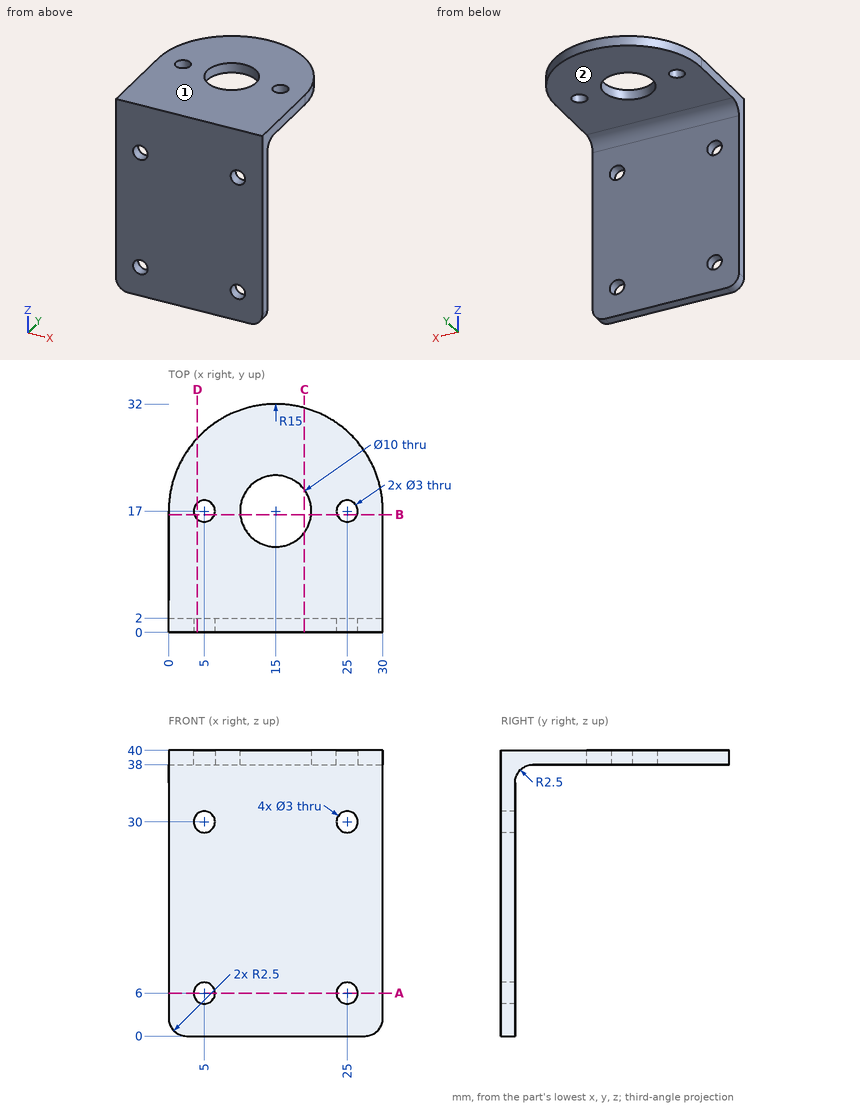
Input: dimensioned drawing with shaded views. Units: mm. Origin: part minimum x, y, z. A direction names the side the tool comes from. Give positions to 0.01 mm unless a question says otherwise; leave off trailing zeros. Loops run counter-clockwise (first coordinate to the right, second up) from the corner with the lowest first, then second, coordinate; pieces in that order, holes last. Notation, with made-up numbers: (4.5, -36.75) - (56.5, -36.75) arc R27 ccw to (56.5, -0.75) - close; hole circle Ø6 at (83, 60.25). An arc over 180 degrees is marked (long way). Answer as CSV lines item,"result". Start each with the question number.
(1) Section query B-B (y = 16.5). Output: boundary loops of the cut face in (x, z), and give its area (3 significant figures).
(2) Pin query (flat end, axial travel): P1, Ø4, axis at x = 4, y = 22, coming from the -Z side. Return the tip coordinate at first contact, or that it passes through.
(3) Reachability of the marked faces 1 and 2 from +Z, -Z, +X, -X, +Y, -Y: full face, straight path, thin tool, end or side. Return the list, or none.
(4) Ray query, line 1 along Z through (x, y) = (5, 1.5); line 2 along Y through (x, z) = (11.5, 8.5); line 3 along Z through (x, y) = (1.5, 5). Return the intervals inside material, ascending. Write a range as [from, to].
(5) Section query A-A (z = 6). Output: boundary loops of the cut face in (x, y), and give its area (3 significant figures).
(6) Section query C-C (x = 19). Output: boundary loops of the cut face in (y, z).
(7) Section query D-D (x = 4). Output: boundary loops of the cut face in (y, z).
Worked answers:
1,outline,"(0, 38) - (3.59, 38) - (3.59, 40) - (0, 40) - close; (6.41, 38) - (10.03, 38) - (10.03, 40) - (6.41, 40) - close; (19.97, 38) - (23.59, 38) - (23.59, 40) - (19.97, 40) - close; (26.41, 38) - (30, 38) - (30, 40) - (26.41, 40) - close"
1,area,"28.8 mm^2"
2,P1,"stops at z = 38"
3,face 1,"+Z, +X, -X, +Y, -Y"
3,face 2,"-Z, +X, -X, +Y"
4,line 1,"z = [0, 4.5], [7.5, 28.5], [31.5, 40]"
4,line 2,"y = [0, 2]"
4,line 3,"z = [38, 40]"
5,outline,"(0, 0) - (3.5, 0) - (3.5, 2) - (0, 2) - close; (6.5, 0) - (23.5, 0) - (23.5, 2) - (6.5, 2) - close; (26.5, 0) - (30, 0) - (30, 2) - (26.5, 2) - close"
5,area,"48.0 mm^2"
6,outline,"(0, 0) - (2, 0) - (2, 35.5) arc R2.5 cw to (4.5, 38) - (14, 38) - (14, 40) - (0, 40) - close; (20, 38) - (31.46, 38) - (31.46, 40) - (20, 40) - close"
7,outline,"(0, 0) - (2, 0) - (2, 4.88) - (0, 4.88) - close; (0, 7.12) - (2, 7.12) - (2, 28.88) - (0, 28.88) - close; (0, 31.12) - (2, 31.12) - (2, 35.5) arc R2.5 cw to (4.5, 38) - (15.88, 38) - (15.88, 40) - (0, 40) - close; (18.12, 38) - (27.2, 38) - (27.2, 40) - (18.12, 40) - close"
